The drawing under review shows one solid part. Ordinate dimensions are in mm from its lowest x, y, z. A direction names the side the tool comes from. Coordinates: 2 decimals unless noted, no trailing zeros. Write each loop counter-clockwise with the first axis right and the second up, starting at its lowest first coordinate (ties: lowest second). Pieces come first, ordered by that corner, then holes. Notation, with made-up numbers: (57.5, 69) - (78.5, 69) arc R25 ccw to (78.5, 106) - close; hole circle Ø9 at (65, 59.25). An arc over 180 degrees is marked (long way). Put each result on its own line as item: value. Start each with the question number.
Item 1: Consider section C-C on z = 6.5. Give the boundary of the cut face in (x, y).
Item 2: Consider section A-A on x = 9. Give the boundary of the cut face in (y, z).
Item 3: To check wall thickness, follow L1, parallel to Z at x = 9, y = 2.5; L2, parallel to Z at x = 9, y = 1.2; L3, parallel to X at y = 0.65, z = 6.5. State the ranges of each line that lie inside material, in increasing order. Write a range as [from, to].
Item 4: Consider section D-D on x = 13. Give the boundary of the cut face in (y, z), then the cut area to 3 significant figures.
Item 5: Machinability: for the marked faces 1, 2, 3, 4 and 5, which of the approach directions +Z, -Z, +X, -X, +Y, -Y give a long, thin tool a straight path to every point of the face, cutting with its end or side? Answer none if there is none.
Item 6: Mouldability with a two-part tool opening along X and no side actions: class the marked faces 6, 7 and 8 as pulls with the +X half, pulls with the -X half, needs draft (parallel to the pull), parting line crosses it, or undercut.
Item 7: For pin 1 (2.5 mm diameter, centred on x = 9, z = 6.5, fed in from -Y); pin 2 (1.6 mm diameter, centred on y = 3, z = 7.5, fed in from -X); pin 3 (2 mm diameter, centred on y = 1, z = 7.5, fed in from -X); pin 4 (1.6 mm diameter, centred on x = 11, y = 2.5, fed in from +Z), all flat-tipped, find the tip position at first contact; note any pin that passes through.
Item 8: Consider section B-B on y = 0.3. Give the boundary of the cut face in (x, z).
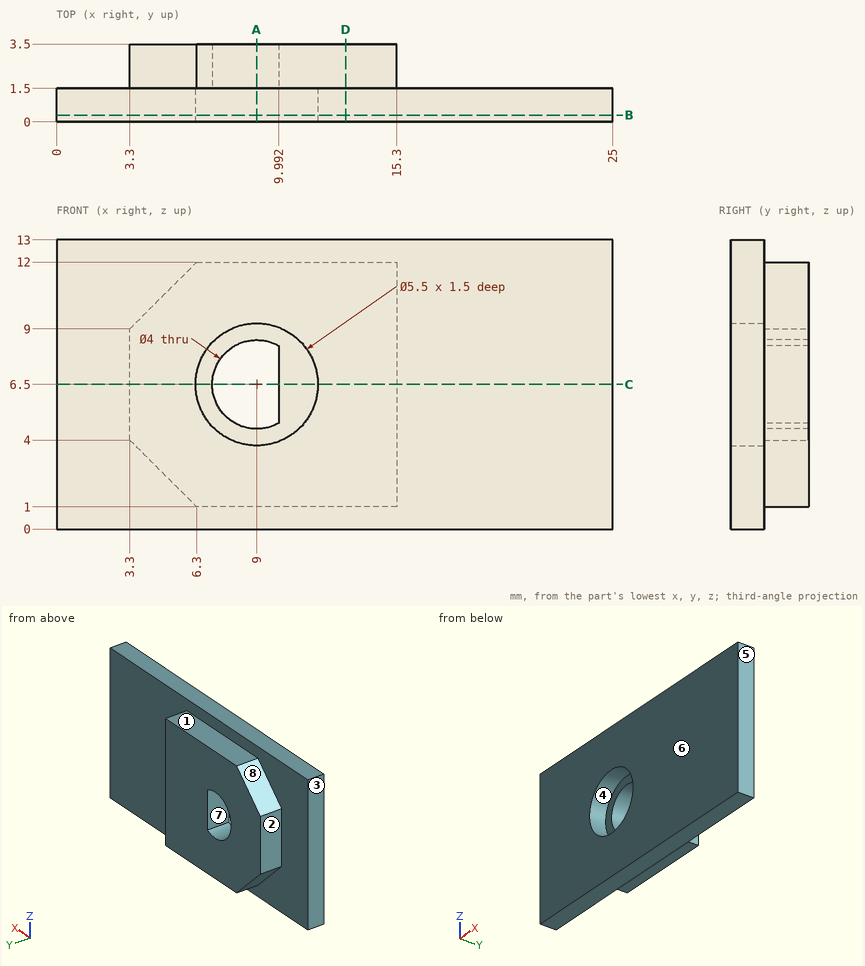
Report:
1. outline: (0, 0) - (6.25, 0) - (6.25, 1.5) - (7, 1.5) - (7, 3.5) - (3.3, 3.5) - (3.3, 1.5) - (0, 1.5) - close; (9.99, 1.5) - (11.75, 1.5) - (11.75, 0) - (25, 0) - (25, 1.5) - (15.3, 1.5) - (15.3, 3.5) - (9.99, 3.5) - close
2. outline: (0, 0) - (1.5, 0) - (1.5, 1) - (3.5, 1) - (3.5, 4.5) - (1.5, 4.5) - (1.5, 3.75) - (0, 3.75) - close; (0, 9.25) - (1.5, 9.25) - (1.5, 8.5) - (3.5, 8.5) - (3.5, 12) - (1.5, 12) - (1.5, 13) - (0, 13) - close
3. L1: [1, 4.5], [8.5, 12]
3. L2: [0, 3.75], [9.25, 13]
3. L3: [0, 6.25], [11.75, 25]
4. outline: (0, 0) - (1.5, 0) - (1.5, 1) - (3.5, 1) - (3.5, 12) - (1.5, 12) - (1.5, 13) - (0, 13) - close
4. area: 41.5 mm²
5. face 1: +Z, +X, -X, +Y
5. face 2: +Z, -Z, -X, +Y
5. face 3: +Z, -Z, -X, +Y, -Y
5. face 4: -Y
5. face 5: +Z, -Z, +X, +Y, -Y
6. face 6: needs draft
6. face 7: undercut
6. face 8: pulls with the -X half
7. pin 1: y = 1.5
7. pin 2: x = 3.3
7. pin 3: x = 0
7. pin 4: z = 12
8. outline: (0, 0) - (25, 0) - (25, 13) - (0, 13) - close; hole circle Ø5.5 at (9, 6.5)
